The model under review builds one solid part; all positions refer to its coordinate system, in mm. A direction names the side the tool comes from. Round coordinates to 2 decimals unless told otherwise and drop trailing zeros. Order: outer loops, then holes, each group sorted by start corner. A loop starts at its lowest first (then second) coordinate and runs counter-clockwise, first axis right, second up. Notation, with made-up numbers: (-4, 56) -> (19, 56) arc R22 ccw to (19, 87) -> close; hole circle Ø9 at (54, 30). An arc over 180 degrees is marked (long way). Use a Markdown table: item, result. Add a question column.
```python
from build123d import *

# Parameters (mm, degrees)
SKETCH1_R           = 37.5
BOSS_EXTRUDE1_DEPTH = 8
FILLET1_R           = 10
BOSS_EXTRUDE3_DEPTH = 77


with BuildPart() as part:
    # Sketch1 → Boss-Extrude1 (new body)
    with BuildSketch(Plane(origin=(0, 0, 0), x_dir=(1, 0, 0), z_dir=(0, 1, 0))):
        with Locations(Location((0, 0, 0), (0, 0, 270))):
            Circle(SKETCH1_R)
    extrude(amount=BOSS_EXTRUDE1_DEPTH)

    # Fillet1
    # the kernel refuses this fillet: 10 mm, written as the material it takes off along each edge
    with BuildSketch(Plane(origin=(0, 8, 0), x_dir=(0, 0, 1), z_dir=(-1, 0, 0))) as fillet1_piece_1:
        with BuildLine():
            CenterArc((27.702041029, -10), FILLET1_R, 11.536959033, 78.463040967)
            Line((27.702041029, 0), (27.702041029, 0.2))
            Line((27.702041029, 0.2), (37.5, 0.2))
            Line((37.5, 0.2), (37.7, 0))
            ThreePointArc((37.7, 0), (37.7, -4), (37.695959179, -7.96))
            Line((37.695959179, -7.96), (37.5, -8))
        make_face()
    revolve(axis=Axis((0, 8, 0), (0, 1, 0)), mode=Mode.SUBTRACT)

    # Sketch3 → Boss-Extrude3 (add)
    with BuildSketch(Plane.XZ):
        with BuildLine():
            Line((-31.557930538, -20.257023971), (-23.752439757, 29.018470077))
            ThreePointArc((-23.752439757, 29.018470077), (-37.038194394, 5.867039803), (-31.557930538, -20.257023971))
        make_face()
        with BuildLine():
            ThreePointArc((37.5, 0), (36.396457433, 9.03038683), (33.150779397, 17.529284794))
            Line((33.150779397, 17.529284794), (26.110331633, -26.916548479))
            ThreePointArc((26.110331633, -26.916548479), (34.535398045, -14.613564996), (37.5, 0))
        make_face()
    extrude(amount=BOSS_EXTRUDE3_DEPTH)


solid = part.part
```
Q1. Add section B-B (y = 3.5). Write out the cut boundary in (x, z).
Q2. Insertion check: pin 1 (4 mm diameter, centred on y = -66.5, z = -7.5, fed in from +X); pin 2 (19.5 mm diameter, centred on x = 9.5, z = 3.5, fed in from -Y); pin 3 (3 mm diameter, centred on y = -24, z = 14, fed in from +X). Each pin has a flat end and moves straight along its axis. Give the tip position at first contact, or say it passes through.
Q3. Add section A-A (y = -9.5). Write out the cut boundary in (x, z).
Q4. Wall thickness on line 1 (X direction, y = -56.5, z = -15.5); line 2 (X direction, y = -32, z = -16.5); line 3 (Y direction, x = -14, z = 3.5): over which ranges is each line inside the solid? List them lowest first. Write a range as [from, to].
Q5. Machinability: for faces 1 (the flat face through (29.68, -37.96, -4.38)), 2 (the cylindrical face through (-36.976, -37.961, 6.244)), 3 (the flat face through (-27.71, -37.96, 4.04)), which of the approach directions +Z, -Z, +X, -X, +Y, -Y give a long, thin tool a straight path to every point of the face, cutting with its end or side? Answer none if there is none.
Report:
| question | item | result |
|---|---|---|
| 1 | outline | circle Ø72.11 at (0, 0) |
| 2 | pin 1 | stops at x = 37.09 |
| 2 | pin 2 | stops at y = 0 |
| 2 | pin 3 | stops at x = 35.36 |
| 3 | outline | (-31.56, -20.26) -> (-23.75, 29.02) arc R37.5 ccw to start; (26.11, -26.92) arc R37.5 ccw to (33.15, 17.53) -> close |
| 4 | line 1 | x = [-34.15, -30.8], [27.92, 34.15] |
| 4 | line 2 | x = [-33.67, -30.96], [27.76, 33.67] |
| 4 | line 3 | y = [0, 8] |
| 5 | face 1 | +Z, -Y |
| 5 | face 2 | -X, +Y, -Y |
| 5 | face 3 | -Z, -Y |
